Here's how the part is built. I have some questions about the finished solid (model axes, mm). A direction names the side the tool comes from. Round coordinates to 2 decimals unless told otherwise and drop trailing zeros. Write each loop counter-clockwise with the first axis right and the second up, starting at its lowest first coordinate (ties: lowest second). Pieces come first, ordered by that corner, then holes. Notation, with made-up numbers: M -10.75,-3.75 L 19.25,-3.75 A24 cw 19.25,8.25 Z; hole C -13,55 d3. An arc over 180 degrees is marked long. Write item = value, one per line. Start each with the question number.
(1) I need wall thicknesses on line 1 along X through (y, z) = (3.75, 0) (1 decimal); line 2 along X through (y, z) = (-10.5, 7.75) (1 decimal); line 3 along Z through (x, y) = (-18.5, 1.75) (3 decimals). Which ranges of each line are inside material? Lowest first, please.
(2) Will these pins go through, and if not, where does the flat tip stop? pin 1 Ø12.5 at (x, y) = (-18, -5.5) entering from -Z (3 decimals); pin 2 Ø0.5 at (y, z) = (5.5, -10) entering from -X; pin 3 Ø3.5 at (x, z) = (5.56, 7.94) entering from -Y; pin 4 Ø12.5 at (x, y) = (-18.5, 4.5) entering from +Z (3 decimals).
(3) I want a section at C-C (y = -8.5). Give the number of separate pieces and of enclosed holes in the cut face, and give its area (3 significant figures).
(4) On a 3-axis mill with a long thin cutter (end or side, diameter ignored), from which of +Z, -Z, +X, -X, +Y, -Y can I reach the whole of each face in a straight line? I mean faces 1 (the flat face through (36.512, 0, 0)), 2 (the flat face through (-14, 0, 9.525)), 3 (the flat face through (0, 0, -10)). Say none if no direction works.
(5) I want a section at A-A (x = 25.4). List the corners of the cut face in (y, z) for me (1 decimal), and give its area (3 significant figures).
(6) If we mould it in two halves opening along Z, with no side actions, what happens to faces 4 (the cylindrical face through (3.866, -0.178, 7.058)), 5 (the flat face through (0, 0, 10)), 6 (the cylindrical face through (28.55, 0.18, 0.41)), 7 (the flat face through (-14, 0, -9.525))? For each: released by +Z, released by -Z, zero draft, split by the parting line, or undercut.
(7) I want a section at B-B (z = 0). List the corners of the cut face in (x, y) for me (1 decimal).
```python
from build123d import *

# Parameters (mm, degrees)
SKETCH1_W               = 28.575
SKETCH1_H               = 19.05
BOSS_EXTRUDE1_DEPTH     = 12.7
SKETCH3_R               = 1.905
CUT_EXTRUDE1_DEPTH      = 46.845504823
CUT_EXTRUDE4_DEPTH      = 41.223628783
CUT_EXTRUDE4_DEPTH_BACK = 41.223628783
SKETCH2_R               = 3.175


with BuildPart() as part:
    # Sketch1 → Boss-Extrude1 (new, symmetric)
    with BuildSketch(Plane(origin=(0, 0, 0), x_dir=(1, 0, 0), z_dir=(0, 1, 0))):
        with Locations((-14.2875, 0)):
            Rectangle(SKETCH1_W, SKETCH1_H)
        Polygon((0, 9.525), (0, -9.525), (0, -11.1125), (36.5125, -11.1125), (36.5125, 11.1125), (0, 11.1125), align=None)
    extrude(amount=BOSS_EXTRUDE1_DEPTH, both=True)

    # Sketch3 → Cut-Extrude1 (cut, through all)
    with BuildSketch(Plane.XZ.offset(12.7)):
        with Locations(Location((5.55625, 7.9375, 0), (0, 0, 270))):
            Circle(SKETCH3_R)
        with Locations(Location((5.55625, -7.9375, 0), (0, 0, 270))):
            Circle(SKETCH3_R)
    extrude(amount=-CUT_EXTRUDE1_DEPTH, mode=Mode.SUBTRACT)

    # Sketch2 → Cut-Extrude4 (cut, two sides: drawn at the far end of the back side and taken through both)
    with BuildSketch(Plane.XZ.offset(-CUT_EXTRUDE4_DEPTH_BACK)):
        with Locations(Location((25.4, 0, 0), (0, 0, 270))):
            Circle(SKETCH2_R)
    extrude(amount=CUT_EXTRUDE4_DEPTH + CUT_EXTRUDE4_DEPTH_BACK, mode=Mode.SUBTRACT)


solid = part.part
```
Returned:
q1.line_1 = -28.6 to 22.2, 28.6 to 36.5
q1.line_2 = -28.6 to 3.7, 7.5 to 36.5
q1.line_3 = -9.525 to 9.525
q2.pin_1 = -9.525
q2.pin_2 = 0
q2.pin_3 = through
q2.pin_4 = 9.525
q3.separate_pieces = 1
q3.enclosed_holes = 3
q3.area = 1,300 mm²
q4.face_1 = +Z, -Z, +X, +Y, -Y
q4.face_2 = +Z, -X, +Y, -Y
q4.face_3 = -Z, -X, +Y, -Y
q5.outline = M -12.7,-11.1 L 12.7,-11.1 L 12.7,-3.2 L -12.7,-3.2 Z; M -12.7,3.2 L 12.7,3.2 L 12.7,11.1 L -12.7,11.1 Z
q5.area = 403 mm²
q6.face_4 = undercut
q6.face_5 = zero draft
q6.face_6 = undercut
q6.face_7 = released by -Z
q7.outline = M -28.6,-12.7 L 22.2,-12.7 L 22.2,12.7 L -28.6,12.7 Z; M 28.6,-12.7 L 36.5,-12.7 L 36.5,12.7 L 28.6,12.7 Z
